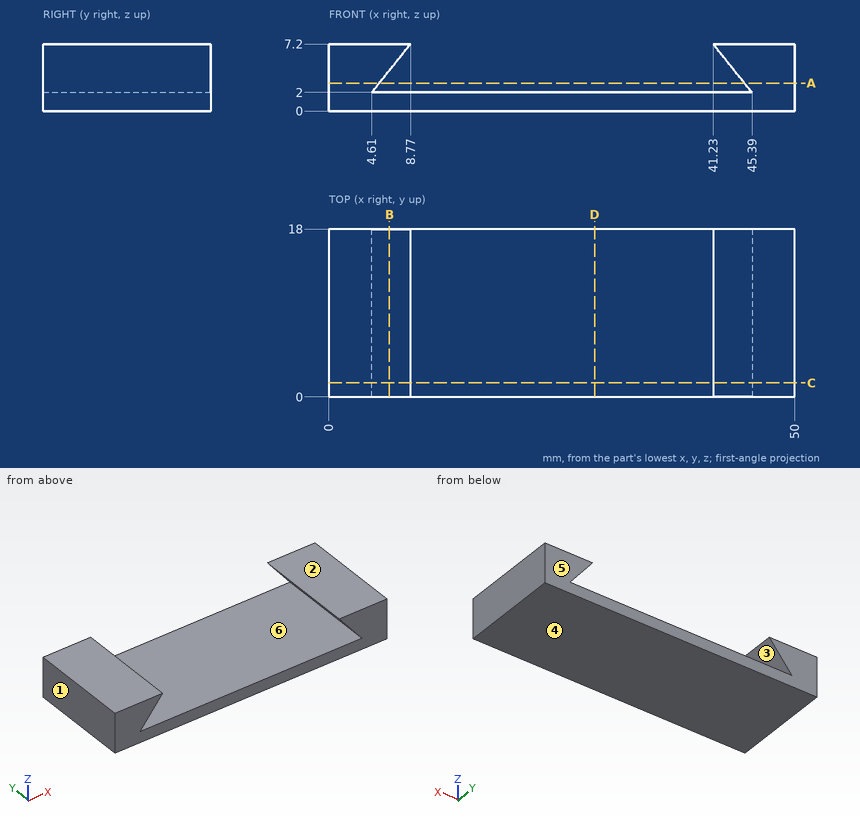
The figure shows three views and two pictorial views of one solid part (mm, origin at its lowest corner). Answer the questions. A direction names the side the tool comes from. Give positions to 0.01 mm unless a question says otherwise; leave off trailing zeros. Loops run counter-clockwise (first coordinate to the right, second up) from the corner with the lowest first, then second, coordinate; pieces in that order, holes last. Notation, with made-up numbers: (-12, -36.75) - (38, -36.75) arc R8 cw to (38, -31.75) - close; hole circle Ø11 at (-15, 6.25). An arc over 180 degrees is marked (long way). Answer in a Markdown table with one row per item.
(1) Section C-C (y = 1.5) is taken. Give the vertices of the cut face in (x, z).
Results list:
| item | result |
|---|---|
| outline | (0, 0) - (50, 0) - (50, 7.2) - (41.23, 7.2) - (45.39, 2) - (4.61, 2) - (8.77, 7.2) - (0, 7.2) - close |
(2) A tool of negligible diameter and unlimited length cuts with its end or side. For the marked faces 5 and 6, from which of +Z, -Z, +X, -X, +Y, -Y can it reach the whole face along a straight path? Write none if from no direction.
Results list:
| item | result |
|---|---|
| face 5 | +Z, -Z, +X, -X, +Y |
| face 6 | +Y, -Y |
(3) Section B-B (x = 6.5) is taken. Give the vertices of the cut face in (y, z), and give its area (3 significant figures).
Results list:
| item | result |
|---|---|
| outline | (0, 0) - (18, 0) - (18, 2) - (0, 2) - close; (0, 4.36) - (18, 4.36) - (18, 7.2) - (0, 7.2) - close |
| area | 87.1 mm² |
(4) Section D-D (x = 28.5) is taken. Give the vertices of the cut face in (y, z).
Results list:
| item | result |
|---|---|
| outline | (0, 0) - (18, 0) - (18, 2) - (0, 2) - close |
(5) Consider L1, parallel to Z at x = 22.5, y = 9.75; L2, parallel to X at y = 15.5, z = 3.5; L3, parallel to X at y = 10.5, z = 4.75. Determine where each line is inside the solid, lowest interval first. Write a range as [from, to].
Results list:
| item | result |
|---|---|
| L1 | z = [0, 2] |
| L2 | x = [0, 5.81], [44.19, 50] |
| L3 | x = [0, 6.81], [43.19, 50] |
(6) Section A-A (z = 3) is taken. Give the vertices of the cut face in (x, y), and give its area (3 significant figures).
Results list:
| item | result |
|---|---|
| outline | (0, 0) - (5.41, 0) - (5.41, 18) - (0, 18) - close; (44.59, 0) - (50, 0) - (50, 18) - (44.59, 18) - close |
| area | 195 mm² |
(7) For a pull along Z with two mould halves and no side action, classify the marked faces 1, 2, 3 and 4 as pulls with the +Z half, pulls with the -Z half, needs draft (parallel to the pull), parting line crosses it, or undercut.
Results list:
| item | result |
|---|---|
| face 1 | needs draft |
| face 2 | pulls with the +Z half |
| face 3 | undercut |
| face 4 | pulls with the -Z half |
